Input: part model. Units: mm. Frame: model coordinates. Coordinates: 2 decimals unless noted, no trailing zeros. Write each loop counter-clockwise with the first axis right and the second up, starting at its lowest first coordinate (ties: lowest second). Pieces come first, ordered by that corner, then holes. Notation, with made-up numbers: (1, 72) -> (34, 72) arc R7 ccw to (34, 83) -> close; hole circle Ø9 at (73, -22). An arc over 180 degrees is marked (long way). Use one line per item in the form item = value. Start each with the question number.
(1) Cut plane D-D on y = 6.5. Return the cut outline in (x, z).
(2) Cut plane B-B on x = -3. State how many separate pieces and enclosed holes the cut face has, plus the area to 3 significant figures.
(3) Ray query, line 1 along Y through (x, z) = (1.5, -2.25); line 2 along Y through (x, z) = (-2.25, -1.25); line 3 along X through (y, z) = (0.75, 1.5). Return the intervals inside material, ascending.
(4) Cut plane A-A on y = 2.5. Return the cut outline in (x, z) (3 decimals).
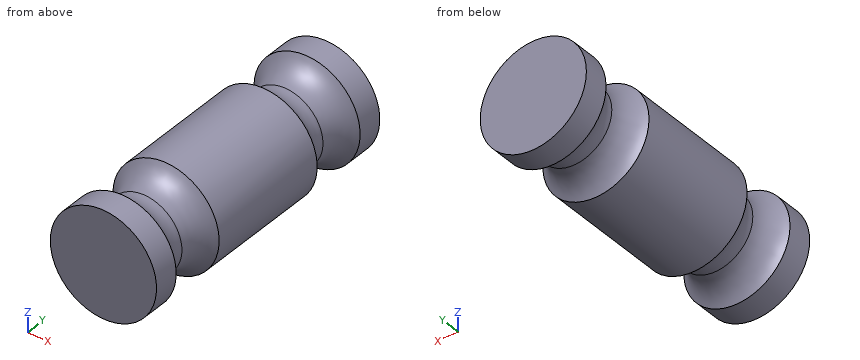
```python
from build123d import *

# Parameters (mm, degrees)
F0_W   = 2.2352
F0_H   = 1.524
F0_W_2 = 0.9398
F0_H_2 = 7.5946


# Not quite as in the source:
# - a feature names something its author has since deleted; it is built from what else it names


with BuildPart() as f1:
    # F0 (on Top) → F1 (revolve)
    with BuildSketch(Plane.XY):
        with Locations((1.1176, 7.8867)):
            Rectangle(F0_W, F0_H)
        Polygon((2.2352, 7.1247), (0, 7.1247), (0, 3.7973), (2.2352, 3.7973), (2.2352, 5.4609999998), align=None)
        with Locations((-2.7051, 7.8867)):
            Rectangle(F0_W_2, F0_H)
        with Locations((1.1176, 0)):
            Rectangle(F0_W, F0_H_2)
        with BuildLine():
            Line((-2.2352, 5.461), (-2.2352, 7.1247))
            Line((-2.2352, 7.1247), (-3.175, 7.1247))
            ThreePointArc((-3.175, 7.1247), (-2.4863911938, 6.4163954325), (-2.2352, 5.461))
        make_face()
        Polygon((2.2352, -3.7973), (0, -3.7973), (0, -7.1247), (2.2352, -7.1247), (2.2352, -5.4610000002), align=None)
        with BuildLine():
            Line((-3.175, 3.7973), (-2.2352, 3.7973))
            Line((-2.2352, 3.7973), (-2.2352, 5.461))
            ThreePointArc((-2.2352, 5.461), (-2.4863911938, 4.5056045675), (-3.175, 3.7973))
        make_face()
        with Locations((-2.7051, 0)):
            Rectangle(F0_W_2, F0_H_2)
        with Locations((1.1176, -7.8867)):
            Rectangle(F0_W, F0_H)
        with BuildLine():
            Line((-2.2352, -5.461), (-2.2352, -3.7973))
            Line((-2.2352, -3.7973), (-3.175, -3.7973))
            ThreePointArc((-3.175, -3.7973), (-2.4863911938, -4.5056045675), (-2.2352, -5.461))
        make_face()
        with Locations((-2.7051, -7.8867)):
            Rectangle(F0_W_2, F0_H)
        with BuildLine():
            Line((-3.175, -7.1247), (-2.2352, -7.1247))
            Line((-2.2352, -7.1247), (-2.2352, -5.461))
            ThreePointArc((-2.2352, -5.461), (-2.4863911938, -6.4163954325), (-3.175, -7.1247))
        make_face()
        with Locations((2.7051, -7.8867)):
            Rectangle(F0_W_2, F0_H)
    revolve(axis=Axis((0, 0, 0), (0, 1, 0)))


solid = f1.part
```
Values:
q1.outline = circle Ø5.07 at (0, 0)
q2.separate_pieces = 3
q2.enclosed_holes = 0
q2.area = 22.8 mm2
q3.line_1 = -8.65 to -6.73, -4.2 to 4.2, 6.73 to 8.65
q3.line_2 = -8.65 to -6.56, -4.37 to 4.37, 6.56 to 8.65
q3.line_3 = -2.8 to 2.8
q4.outline = circle Ø6.35 at (0, 0)
